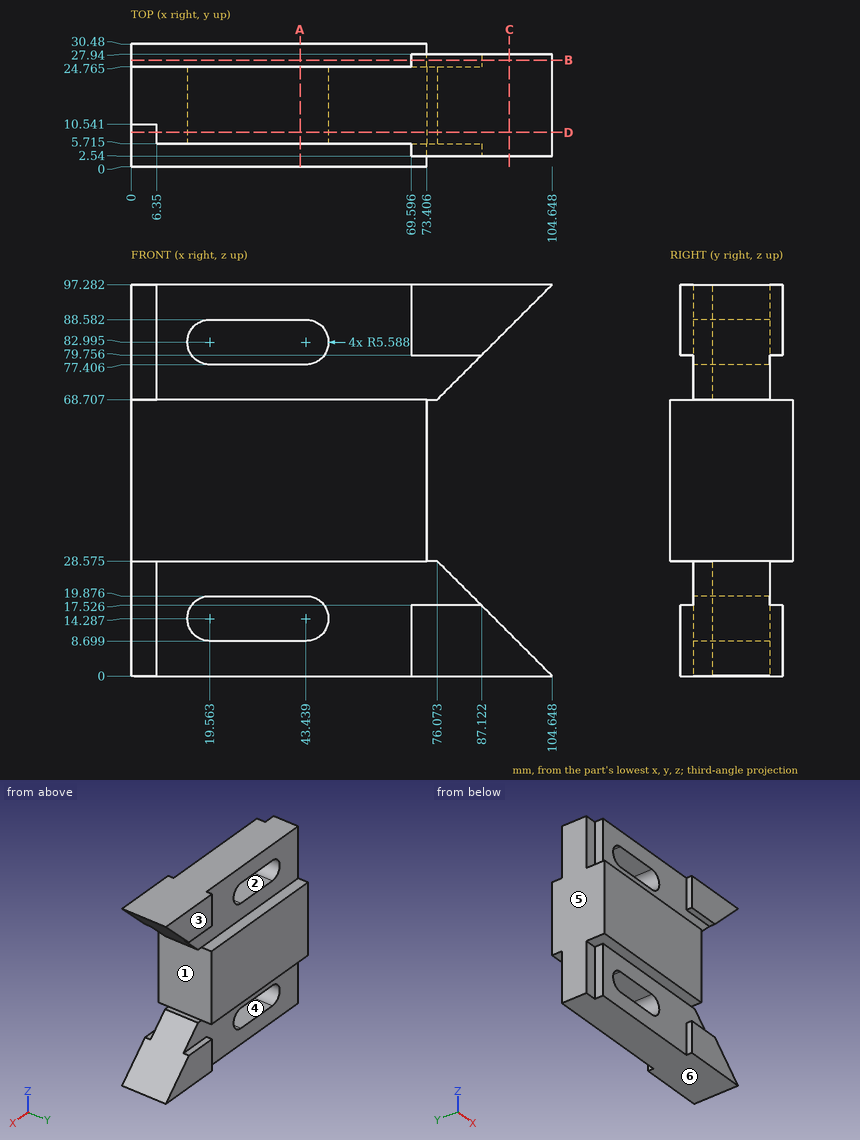
Drawing for the job (mm, zero at the part's lowest x, y, z). A direction names the side the tool comes from. Give positions to 0.01 mm unless a question says otherwise; leave off trailing zeros. Order: outer loops, then holes, each group sorted by start corner. A loop starts at its lowest first (then second) coordinate and runs counter-clockwise, first axis right, second up. Notation, with made-up numbers: (26, 58) - (51, 58) arc R13 ccw to (51, 75) - close; hole circle Ø9 at (11.25, 71.5). An arc over 180 degrees is marked (long way). Use one line per item in the form item = value.
Item 1: Two-plate mould, pull along Z, no slides. Class the marked faces 4, 5 and 6: released by +Z, released by -Z, zero draft, split by the parting line, or undercut.
Solution:
face_4 = undercut
face_5 = zero draft
face_6 = released by -Z
Item 2: Slice it at B-B on y = 26.5. Give the cut face in (x, z) (1 decimal).
Solution:
outline = (0, 28.6) - (73.4, 28.6) - (73.4, 68.7) - (0, 68.7) - close; (69.6, 0) - (104.6, 0) - (87.1, 17.5) - (69.6, 17.5) - close; (69.6, 79.8) - (87.1, 79.8) - (104.6, 97.3) - (69.6, 97.3) - close
Item 3: Pin check, flat tips, straight feed: pin 1 Ø4 at (y, z) = (10, 44.5) entering from +X; pin 2 Ø10 at (x, y) = (83, 21.5) entering from -Z; pin 3 Ø5.5 at (x, z) = (90.5, 11) entering from +Y; pin 4 Ø8.5 at (x, z) = (28.5, 18.5) entering from -Y (1 decimal). Stop position of each tip, or through.
Solution:
pin_1 = 73.41
pin_2 = 0
pin_3 = 27.94
pin_4 = 5.7
Item 4: Which spindle directions (+Z, -Z, +X, -X, +Y, -Y) get a long thin tool onto all of the face, cutting with end or side? Do the marked faces 1, 2 and 3. Say none if no direction does.
Solution:
face_1 = +X, +Y, -Y
face_2 = +Y, -Y
face_3 = +Z, +X, -X, +Y
Item 5: Probe probe 1 along X at (y, z) = (19, 56) (1 decimal); probe 2 along Z at (x, y) = (16.5, 27) (1 decimal); probe 3 along X at (y, z) = (19, 84) (1 decimal). List the from-to ranges inside material, lowest first. Write a range as from..to.
Solution:
probe_1 = 0..73.4
probe_2 = 28.6..68.7
probe_3 = 0..14.1, 48.9..91.4
Item 6: Slice it at A-A on x = 42. Give the cut face in (y, z) (1 decimal), and give its area (3 significant figures).
Solution:
outline = (0, 28.6) - (5.7, 28.6) - (5.7, 19.9) - (24.8, 19.9) - (24.8, 28.6) - (30.5, 28.6) - (30.5, 68.7) - (24.8, 68.7) - (24.8, 77.4) - (5.7, 77.4) - (5.7, 68.7) - (0, 68.7) - close; (5.7, 0) - (24.8, 0) - (24.8, 8.7) - (5.7, 8.7) - close; (5.7, 88.6) - (24.8, 88.6) - (24.8, 97.3) - (5.7, 97.3) - close
area = 1,890 mm2
Item 7: Slice it at D-D on y = 8.5. Count the separate pieces of the cut face and the enclosed holes in it, and give its area (3 significant figures).
Solution:
separate_pieces = 1
enclosed_holes = 2
area = 7,020 mm2
Item 8: Slice it at C-C on x = 94. Give the cut face in (y, z) (1 decimal).
Solution:
outline = (2.5, 0) - (27.9, 0) - (27.9, 10.6) - (2.5, 10.6) - close; (2.5, 86.6) - (27.9, 86.6) - (27.9, 97.3) - (2.5, 97.3) - close
